```python
from build123d import *

# Parameters (mm, degrees)
MODEL_R                 = 1.5
SALIENTE_EXTRUIR1_DEPTH = 3


with BuildPart() as part:
    # Model → Saliente-Extruir1 (new body)
    with BuildSketch(Plane.XY):
        with BuildLine():
            Line((174.227054575, 213.178720063), (174.227054575, 204.178720063))
            ThreePointArc((174.227054575, 204.178720063), (174.569596678, 202.456644617), (175.545074059, 200.996739548))
            Line((175.545074059, 200.996739548), (184.545074059, 191.996739548))
            ThreePointArc((184.545074059, 191.996739548), (187.727054575, 190.678720063), (190.90903509, 191.996739548))
            Line((190.90903509, 191.996739548), (199.90903509, 200.996739548))
            ThreePointArc((199.90903509, 200.996739548), (200.884512471, 202.456644617), (201.227054575, 204.178720063))
            Line((201.227054575, 204.178720063), (201.227054575, 217.678720063))
            Line((201.227054575, 217.678720063), (174.227054575, 217.678720063))
            Line((174.227054575, 217.678720063), (174.227054575, 213.178720063))
        make_face()
        with Locations((187.727054575, 204.178720063)):
            Circle(MODEL_R, mode=Mode.SUBTRACT)
        with Locations((178.727054575, 204.178720063)):
            Circle(MODEL_R, mode=Mode.SUBTRACT)
        with Locations((187.727054575, 213.178720063)):
            Circle(MODEL_R, mode=Mode.SUBTRACT)
        with Locations((178.727054575, 213.178720063)):
            Circle(MODEL_R, mode=Mode.SUBTRACT)
        with Locations((196.727054575, 213.178720063)):
            Circle(MODEL_R, mode=Mode.SUBTRACT)
        with Locations((187.727054575, 195.178720063)):
            Circle(MODEL_R, mode=Mode.SUBTRACT)
        with Locations((196.727054575, 204.178720063)):
            Circle(MODEL_R, mode=Mode.SUBTRACT)
    extrude(amount=SALIENTE_EXTRUIR1_DEPTH)


solid = part.part
```
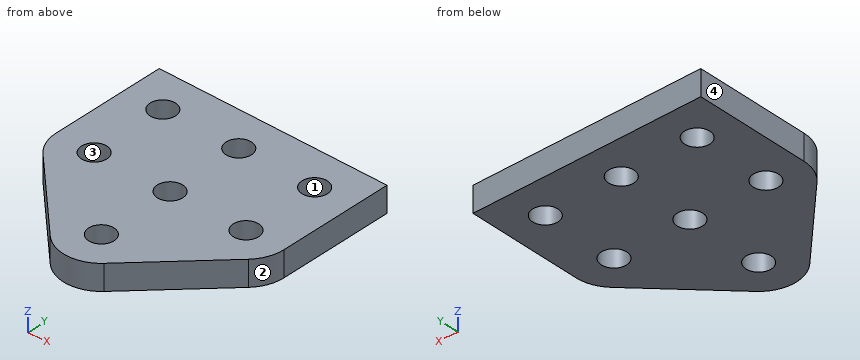
The model under review builds one solid part; all positions refer to its coordinate system, in mm. Face numbers are marked on the shaded views. Round coordinates to 2 decimals unless told otherwise and drop trailing zeros. Loops run counter-clockwise (first coordinate to the right, second up) from the corner with the lowest first, then second, coordinate; pieces in that order, holes last.
1) The part is to be moulded in two halves that separate along Y. For the marked faces 1, 2, 3 and 4, say which applies: pulls with the +Y half, pulls with the -Y half, needs draft (parallel to the pull), parting line crosses it, or undercut.
Values follow:
face 1: undercut
face 2: pulls with the -Y half
face 3: undercut
face 4: needs draft
2) Wall thickness on line 1 along Y through (x, z) = (188, 2.85); line 2 along X through (y, z) = (204.75, 2.1); line 3 along Y through (x, z) = (197, 1.85): over which ranges is each line inside the solid? List them lowest first.
Values follow:
line 1: y = 190.69 to 193.7, 196.65 to 202.7, 205.65 to 211.7, 214.65 to 217.68
line 2: x = 174.23 to 177.34, 180.11 to 186.34, 189.11 to 195.34, 198.11 to 201.23
line 3: y = 198.09 to 202.7, 205.65 to 211.7, 214.65 to 217.68
3) Consider section A-A on x = 187. State the section outline as (y, z) points, then the cut area to 3 significant figures.
Values follow:
outline: (190.74, 0) - (193.87, 0) - (193.87, 3) - (190.74, 3) - close; (196.49, 0) - (202.87, 0) - (202.87, 3) - (196.49, 3) - close; (205.49, 0) - (211.87, 0) - (211.87, 3) - (205.49, 3) - close; (214.49, 0) - (217.68, 0) - (217.68, 3) - (214.49, 3) - close
area: 57.2 mm2
4) Consider section B-B on z = 1.35. State the section outline as (x, y) points.
Values follow:
outline: (174.23, 204.18) arc R4.5 ccw to (175.55, 201) - (184.55, 192) arc R4.5 ccw to (190.91, 192) - (199.91, 201) arc R4.5 ccw to (201.23, 204.18) - (201.23, 217.68) - (174.23, 217.68) - close; hole circle Ø3 at (178.73, 204.18); hole circle Ø3 at (178.73, 213.18); hole circle Ø3 at (187.73, 195.18); hole circle Ø3 at (187.73, 204.18); hole circle Ø3 at (187.73, 213.18); hole circle Ø3 at (196.73, 204.18); hole circle Ø3 at (196.73, 213.18)
5) Clearance check with flat-ended pins moving along their axes: P1, Ø3.5, axis at x = 196.73, y = 204.18, coming from the -Z side; P2, Ø1.5, axis at x = 196, z = 2, coming from the -Y side. State where each tip first meets the part, or that it passes through.
Values follow:
P1: stops at z = 0
P2: stops at y = 196.34
6) Consider section D-D on y = 198.5. State the section outline as (x, z) points, then the cut area to 3 significant figures.
Values follow:
outline: (178.04, 0) - (197.41, 0) - (197.41, 3) - (178.04, 3) - close
area: 58.1 mm2
7) Consider section C-C on x = 179.5. State the section outline as (y, z) points.
Values follow:
outline: (197.04, 0) - (202.89, 0) - (202.89, 3) - (197.04, 3) - close; (205.46, 0) - (211.89, 0) - (211.89, 3) - (205.46, 3) - close; (214.46, 0) - (217.68, 0) - (217.68, 3) - (214.46, 3) - close
